For this review, take the finished solid that the model builds, in its own axes (mm). A direction names the side the tool comes from. Give positions to 0.01 mm unless a question says otherwise; leave off trailing zeros. Write each loop counter-clockwise with the first axis right and the second up, starting at its lowest first coordinate (ties: lowest second). Pieces come first, ordered by that corner, then holes.
Q1. Mouldability with a two-part tool opening along Z and no side actions: class faces 1 (the cylindrical face through (0, -3, 0)), 2 (the flat face through (-25, 3, 38)), 3 (the cylindrical face through (0.168, -2.475, -5.466)) as released by +Z, released by -Z, zero draft, split by the parting line, or undercut.
Q2. We need section C-C (y = -1). Write out the cut boundary in (x, z), then the cut area to 3 significant figures.
Q3. We need section D-D (z = 37.5). Write out the cut boundary in (x, y).
Q4. For line 1 (Y direction, x = 6, z = 0); line 2 (Y direction, x = -0.5, z = 40); line 3 (Y direction, x = 3.5, z = 53), list the stretches that pass through material, from the lowest coordinate up.
Q5. We need section A-A (x = 9). Write out the cut boundary in (y, z).
Q6. Machinability: for faces 4 (the flat face through (-19, 2, 7.5)), 5 (the flat face through (0, 5, 59)), 6 (the flat face through (25, 3, 38)), 7 (the flat face through (0, 0, 41)), 8 (the flat face through (18, 2, 7.5)), which of the approach directions +Z, -Z, +X, -X, +Y, -Y give a long, thin tool a straight path to every point of the face, cutting with its end or side? Answer none if there is none.
Q7. We need section B-B (z = 1). Write out the cut boundary in (x, y).
Q8. Insertion check: P1, Ø5, axis at y = 0, z = 0, coming from the +X side; P2, Ø4, axis at x = -16.5, y = 4, coming from the -Z side; P3, Ø5, axis at x = 3, y = -3, coming from the -Z side; P4, Ø8, axis at x = -2.5, z = 33, coming from the -Y side. Each pin has a flat end and moves straight along its axis. Give the tip position at first contact, or say it passes through.
```python
from build123d import *

# Parameters (mm, degrees)
F0_R     = 3
F1_DEPTH = 25
F2_W     = 13
F2_H     = 15
F3_DEPTH = 12.5
F4_W     = 1
F4_H     = 16
F5_DEPTH = 30
F6_R     = 14


with BuildPart() as f1:
    # F0 (on Right) → F1 (new body, symmetric)
    with BuildSketch(Plane.YZ):
        with BuildLine():
            Line((-3e-06, 67.431174), (-3e-06, 6))
            ThreePointArc((-3e-06, 6), (-4.242643, -4.242641), (5.999997, 0))
            Line((5.999997, 0), (5.999997, 67.431174))
            Line((5.999997, 67.431174), (-3e-06, 67.431174))
        make_face()
        with Locations((-3e-06, 0)):
            Circle(F0_R, mode=Mode.SUBTRACT)
    extrude(amount=F1_DEPTH, both=True)

    # F2 (on Front) → F3 (cut, symmetric)
    with BuildSketch(Plane.XZ):
        with Locations((-18.5, 0)):
            Rectangle(F2_W, F2_H)
        with Locations((18.5, 0)):
            Rectangle(F2_W, F2_H)
    extrude(amount=F3_DEPTH, both=True, mode=Mode.SUBTRACT)

    # F4 (on Right) → F5 (cut, symmetric)
    with BuildSketch(Plane.YZ):
        with Locations((5.499997, 59.431174)):
            Rectangle(F4_W, F4_H)
    extrude(amount=F5_DEPTH, both=True, mode=Mode.SUBTRACT)

    # F6
    f6_edges = [f1.edges().sort_by_distance(p)[0] for p in [
        (0, -3e-06, 6),
    ]]
    fillet(f6_edges, radius=F6_R)


solid = f1.part
```
Computed:
1. face 1: undercut
1. face 2: zero draft
1. face 3: split by the parting line
2. outline: (-25, 7.5) - (-12, 7.5) - (-12, 2.83) - (12, 2.83) - (12, 7.5) - (25, 7.5) - (25, 9.09) - (-25, 9.09) - close; (-12, -5.92) - (12, -5.92) - (12, -2.83) - (-12, -2.83) - close
2. area: 266 mm2
3. outline: (-25, 0) - (25, 0) - (25, 6) - (-25, 6) - close
4. line 1: y = -6 to -3, 3 to 6
4. line 2: y = 0 to 6
4. line 3: y = 0 to 5
5. outline: (-4.2, 4.28) arc R6 ccw (long way) to (6, 0) - (6, 51.43) - (5, 51.43) - (5, 67.43) - (0, 67.43) - (0, 14.28) arc R14 cw to start; hole circle Ø6 at (0, 0)
6. face 4: -Z, -X, +Y, -Y
6. face 5: +Z, +X, -X, +Y
6. face 6: +Z, -Z, +X, +Y, -Y
6. face 7: +Z, +X, -X, -Y
6. face 8: -Z, +X, +Y, -Y
7. outline: (-12, -5.92) - (12, -5.92) - (12, -2.83) - (-12, -2.83) - close; (-12, 2.83) - (12, 2.83) - (12, 6) - (-12, 6) - close
8. P1: passes through
8. P2: stops at z = 7.5
8. P3: stops at z = -5.98
8. P4: stops at y = 0
